Work out the finished part from the listing and answer in its coordinate system (mm). A direction names the side the tool comes from. Give positions to 0.01 mm unless a question says otherwise; leave off trailing zeros. Order: outer loops, then holes, each group sorted by start corner. A loop starts at its lowest first (then second) coordinate and runs counter-clockwise, first axis right, second up. Notation, with made-up numbers: (22, 38.5) -> (64, 38.5) arc R21 ccw to (64, 56.5) -> close; hole circle Ø8 at (-19, 20). An arc over 180 degrees is marked (long way). Answer as CSV lines item,"result". Start each with the question number.
1. A cutting plane is placed at B-B (z = -27.5). Give the vertices of the cut face in (x, y).
2. For a pull along X with two mould halves and no side action, classify faces 5 (the flat face through (-9, -13, -25.323)), 6 (the flat face through (45.227, -13, -19)), 7 (the flat face through (33, -13, -12.317)) as released by +X, released by -X, zero draft, split by the parting line, or undercut.
3. Find the intervals of material crossed by L1, parallel to Z at x = 41.5, y = -2; L2, parallel to Z at x = -23, y = -4; L3, parallel to X at y = -6.25, z = -11.5, in increasing order.
4. Flat-ended cylindrical pins translate along their axes: pin 1 (6 mm diameter, centred on x = -35, y = -3, fed in from -Z); pin 2 (1 mm diameter, centred on y = -18.5, z = -6, fed in from -X); pin 3 (8 mm diameter, centred on y = -16, z = 1, fed in from +X); pin 4 (3 mm diameter, centred on x = 7, z = -14.5, fed in from +Y). Find the tip coordinate at first contact, or state that the pin passes through.
5. A cutting plane is placed at C-C (x = 11). Give the vertices of the cut face in (y, z).
6. A cutting plane is placed at D-D (z = 3). Give the vertices of the cut face in (x, y).
7. A cutting plane is placed at A-A (y = -13.75). Give the vertices of the cut face in (x, z).
8. For faces 1 (the flat face through (-8, -13, 5.814)), 2 (the flat face through (-59.73, -12.522, -25.423)), 3 (the flat face through (-50, -13, -7.981)), 4 (the flat face through (43, -13, -25.323)), determine the directions among +Z, -Z, +X, -X, +Y, -Y from which every point of the face is accessible in a straight line to the end or side of a thin tool.
from build123d import *

# Parameters (mm, degrees)
F1_DEPTH = 25.4


with BuildPart() as f1:
    # F0 (on Front) → F1 (new body)
    with BuildSketch(Plane.XZ):
        with BuildLine():
            ThreePointArc((26.2159302875, -25.3233611584), (33.7973274291, -17.7419640168), (41.3787245706, -25.3233611584))
            Line((41.3787245706, -25.3233611584), (45.227330178, -25.3233611584))
            Line((45.227330178, -25.3233611584), (45.227330178, -12.3168108985))
            Line((45.227330178, -12.3168108985), (19.6083635092, -12.3168108985))
            Line((19.6083635092, -12.3168108985), (8.9666387066, 5.8135343716))
            Line((8.9666387066, 5.8135343716), (-25.5204308778, 5.8135343716))
            Line((-25.5204308778, 5.8135343716), (-38.9211215079, -7.9812929034))
            Line((-38.9211215079, -7.9812929034), (-60.9928481281, -16.7508628219))
            Line((-60.9928481281, -16.7508628219), (-60.9928481281, -25.5204327404))
            Line((-60.9928481281, -25.5204327404), (-58.4309473634, -25.3233611584))
            Line((-58.4309473634, -25.3233611584), (-56.5701552345, -25.3233611584))
            ThreePointArc((-56.5701552345, -25.3233611584), (-50.1540526748, -18.9072585986), (-43.737950115, -25.3233611584))
            Line((-43.737950115, -25.3233611584), (26.2159302875, -25.3233611584))
        make_face()
        with BuildLine():
            ThreePointArc((26.2159302875, -25.3233611584), (33.7973274291, -32.9047582999), (41.3787245706, -25.3233611584))
            Line((41.3787245706, -25.3233611584), (26.2159302875, -25.3233611584))
        make_face()
        with BuildLine():
            Line((26.2159302875, -25.3233611584), (41.3787245706, -25.3233611584))
            ThreePointArc((41.3787245706, -25.3233611584), (33.7973274291, -17.7419640168), (26.2159302875, -25.3233611584))
        make_face()
        with BuildLine():
            ThreePointArc((-56.5701552345, -25.3233611584), (-50.1540526748, -31.7394637181), (-43.737950115, -25.3233611584))
            Line((-43.737950115, -25.3233611584), (-56.5701552345, -25.3233611584))
        make_face()
        with BuildLine():
            Line((-56.5701552345, -25.3233611584), (-43.737950115, -25.3233611584))
            ThreePointArc((-43.737950115, -25.3233611584), (-50.1540526748, -18.9072585986), (-56.5701552345, -25.3233611584))
        make_face()
        Polygon((-60.9928481281, -16.7508628219), (-38.9211215079, -7.9812929034), (-60.9928481281, -7.9812929034), align=None)
    extrude(amount=F1_DEPTH)


solid = f1.part
Answer sheet:
1,outline,"(-56.19, -25.4) -> (-44.12, -25.4) -> (-44.12, 0) -> (-56.19, 0) -> close; (26.54, -25.4) -> (41.06, -25.4) -> (41.06, 0) -> (26.54, 0) -> close"
2,face 5,"undercut"
2,face 6,"released by +X"
2,face 7,"zero draft"
3,L1,"z = -25.32 to -12.32"
3,L2,"z = -25.32 to 5.81"
3,L3,"x = -60.99 to 19.13"
4,pin 1,"stops at z = -25.32"
4,pin 2,"stops at x = -37.48"
4,pin 3,"stops at x = 14.14"
4,pin 4,"stops at y = 0"
5,outline,"(-25.4, -25.32) -> (0, -25.32) -> (0, 2.35) -> (-25.4, 2.35) -> close"
6,outline,"(-28.25, -25.4) -> (10.62, -25.4) -> (10.62, 0) -> (-28.25, 0) -> close"
7,outline,"(-60.99, -25.52) -> (-58.43, -25.32) -> (-56.57, -25.32) arc R6.42 ccw to (-43.74, -25.32) -> (26.22, -25.32) arc R7.58 ccw to (41.38, -25.32) -> (45.23, -25.32) -> (45.23, -12.32) -> (19.61, -12.32) -> (8.97, 5.81) -> (-25.52, 5.81) -> (-38.92, -7.98) -> (-60.99, -7.98) -> close"
8,face 1,"+Z, +X, -X, +Y, -Y"
8,face 2,"-Z, +Y, -Y"
8,face 3,"+Z, -X, +Y, -Y"
8,face 4,"-Z, +X, +Y, -Y"
